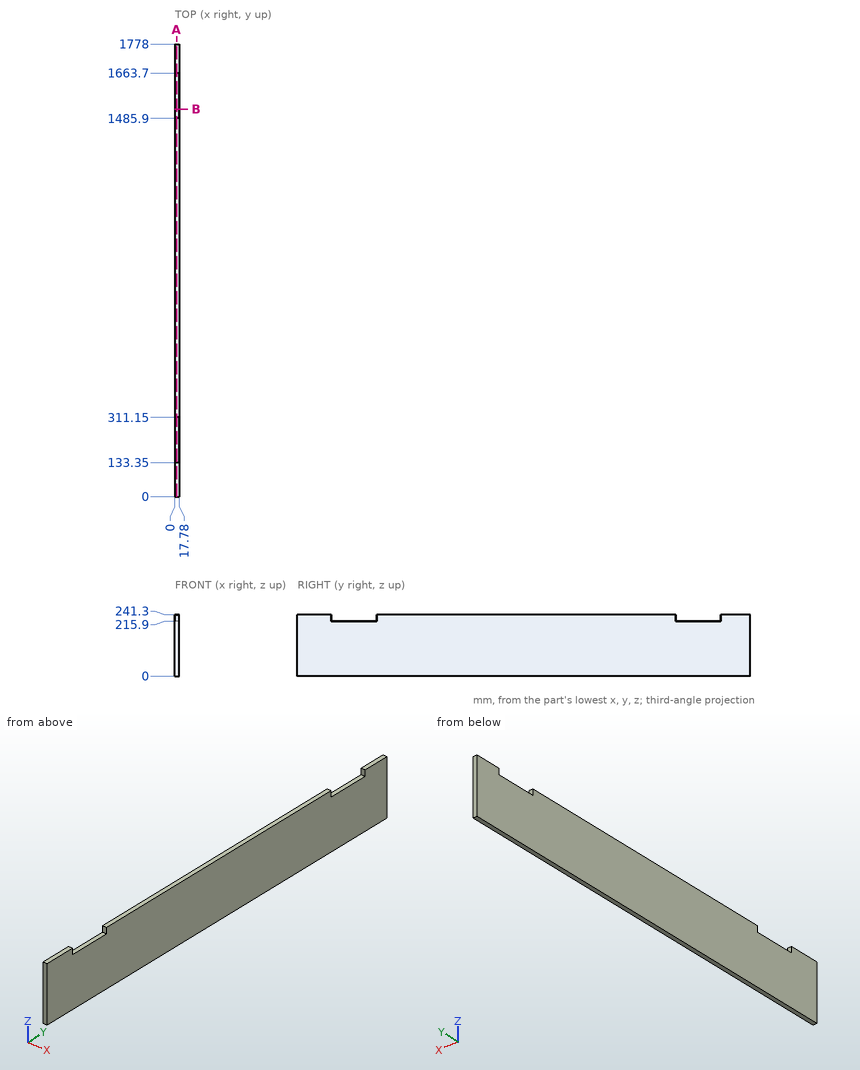
Could you check a few things on this drawing? It's one solid part, dimensions in mm from its lowest x, y, z. Give positions to 0.01 mm unless a question says otherwise; leave off trailing zeros. Write each loop counter-clockwise with the first axis right and the second up, starting at its lowest first coordinate (ties: lowest second). Pieces come first, ordered by that corner, then holes. Notation, with made-up numbers: (71.25, -6) -> (127.25, -6) arc R28 cw to (127.25, 18) -> close; hole circle Ø1 at (-5.5, -33.75). An arc over 180 degrees is marked (long way). Answer as a JSON object with one key per item and string values.
Q1. Suppose I cut it at B-B on y = 1522. Write out the boundary of the cut face in (x, z).
Taken from the geometry:
{"outline": "(0, 0) -> (17.78, 0) -> (17.78, 215.9) -> (0, 215.9) -> close"}
Q2. Please list where these lines run through material, in increasing order: L1, parallel to Y at x = 14.5, z = 230; L2, parallel to Z at x = 3, y = 259.5.
Taken from the geometry:
{"L1": "y = 0 to 133.35, 311.15 to 1485.9, 1663.7 to 1778", "L2": "z = 0 to 215.9"}
Q3. Suppose I cut it at A-A on x = 6.75. Write out the boundary of the cut face in (y, z), then the cut area to 3 significant figures.
Taken from the geometry:
{"outline": "(0, 0) -> (1778, 0) -> (1778, 241.3) -> (1663.7, 241.3) -> (1663.7, 215.9) -> (1485.9, 215.9) -> (1485.9, 241.3) -> (311.15, 241.3) -> (311.15, 215.9) -> (133.35, 215.9) -> (133.35, 241.3) -> (0, 241.3) -> close", "area": "420,000 mm²"}
Q4. Will these pins go through, and if not, where does the flat tip stop? pin 1 Ø8 at (x, y) = (10.5, 330) entering from -Z; pin 2 Ø9 at (x, y) = (10, 181.5) entering from +Z.
Taken from the geometry:
{"pin 1": "stops at z = 0", "pin 2": "stops at z = 215.9"}
